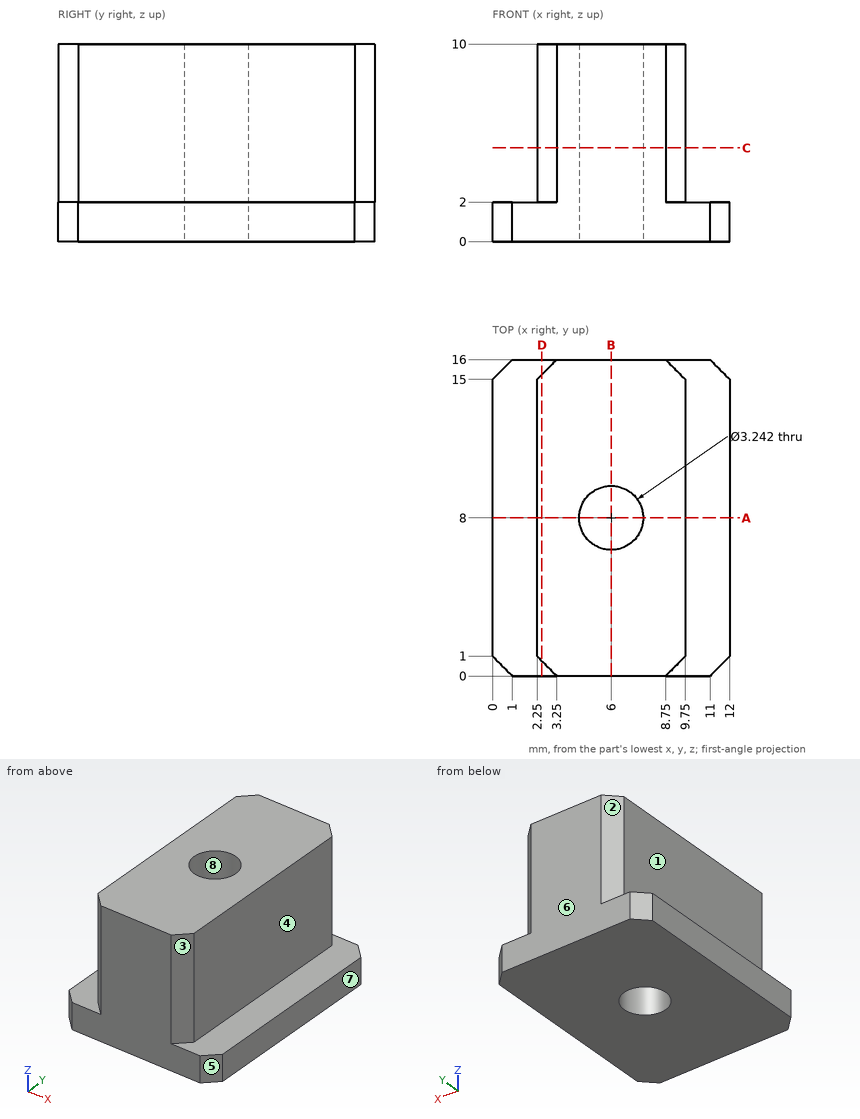
Job drawing, mm, ordinate dimensions from the low corner. One solid piece. A direction names the side the tool comes from. Coordinates: 2 decimals unless noted, no trailing zeros. Write each loop counter-clockwise with the first axis right and the second up, starting at its lowest first coordinate (ties: lowest second). Pieces come first, ordered by that corner, then holes.
Item 1: Slice it at B-B (x = 6). Write the cut outline in (y, z).
Item 2: Probe line 1 (Y direction, x = 6, z = 2.75); line 2 (X direction, y = 8, z = 8.25); line 3 (Z direction, x = 0.75, y = 15). List the from-to ranges inside material, lowest first.
Item 3: Which spindle directions (+Z, -Z, +X, -X, +Y, -Y) get a long thin tool onto all of the face, cutting with end or side? Do the marked faces 1, 2, 3 and 4. Say none if no direction does.
Item 4: Slice it at A-A (y = 8). Write the cut outline in (x, z), and give its area (3 significant figures).
Item 5: Slice it at C-C (z = 4.75). Write the cut outline in (x, y).
Item 6: Pin check, flat tips, straight feed: pin 1 (1.5 mm diameter, centred on y = 8.5, z = 3.5, fed in from -X); pin 2 (2.5 mm diameter, centred on y = 8.5, z = 4, fed in from +X); pin 3 (1 mm diameter, centred on x = 11, y = 9.5, fed in from +Z). Stop position of each tip, or through.
Item 7: Mould opens along Y. For the marked faces 5, 6, 7 and 8 say: released by +Y, released by -Y, zero draft, split by the parting line, or undercut.
Item 8: Slice it at D-D (x = 2.5). Write the cut outline in (y, z).
Results found:
1. outline: (0, 0) - (6.38, 0) - (6.38, 10) - (0, 10) - close; (9.62, 0) - (16, 0) - (16, 10) - (9.62, 10) - close
2. line 1: y = 0 to 6.38, 9.62 to 16
2. line 2: x = 2.25 to 4.38, 7.62 to 9.75
2. line 3: z = 0 to 2
3. face 1: +Z, -X, +Y, -Y
3. face 2: +Z, -X, +Y
3. face 3: +Z, +X, -Y
3. face 4: +Z, +X, +Y, -Y
4. outline: (0, 0) - (4.38, 0) - (4.38, 10) - (2.25, 10) - (2.25, 2) - (0, 2) - close; (7.62, 0) - (12, 0) - (12, 2) - (9.75, 2) - (9.75, 10) - (7.62, 10) - close
4. area: 51.6 mm2
5. outline: (2.25, 1) - (3.25, 0) - (8.75, 0) - (9.75, 1) - (9.75, 15) - (8.75, 16) - (3.25, 16) - (2.25, 15) - close; hole circle Ø3.24 at (6, 8)
6. pin 1: stops at x = 2.25
6. pin 2: stops at x = 9.75
6. pin 3: stops at z = 2
7. face 5: released by -Y
7. face 6: released by +Y
7. face 7: zero draft
7. face 8: undercut
8. outline: (0, 0) - (16, 0) - (16, 2) - (15.25, 2) - (15.25, 10) - (0.75, 10) - (0.75, 2) - (0, 2) - close
